Design review of the part built by this model. Coordinates are the model's own, in mm. Give positions to 0.01 mm unless a question says otherwise; leave off trailing zeros. Loops run counter-clockwise (first coordinate to the right, second up) from the corner with the lowest first, then second, coordinate; pieces in that order, holes last. Notation, with made-up numbers: (21, 4) - (66, 4) arc R19 ccw to (66, 23) - close; hole circle Ø2 at (-19.75, -38). An arc over 180 degrees is marked (long way). Write each question's results on one line, items separated by ' | '.
```python
from build123d import *

# Parameters (mm, degrees)
BOSS_EXTRUDE4_DEPTH  = 3.175
M3_CLEARANCE_HOLE3_D = 3
M3_CLEARANCE_HOLE1_D = 3.1
M3_CLEARANCE_HOLE4_D = 2.95
M3_CLEARANCE_HOLE2_D = 3.1
CUT_EXTRUDE1_DEPTH   = 121.250075364
BOSS_EXTRUDE6_DEPTH  = 3.175
CUT_EXTRUDE3_DEPTH   = 121.250075364
SKETCH25_R           = 1.5
CUT_EXTRUDE4_DEPTH   = 121.250075364


with BuildPart() as part:
    # Sketch1 → Boss-Extrude4 (new body)
    with BuildSketch(Plane(origin=(0, 0, 0), x_dir=(1, 0, 0), z_dir=(0, 1, 0))):
        with BuildLine():
            Line((-62.799553621, 32.496136604), (-73.969425011, 32.691107434))
            Line((-73.969425011, 32.691107434), (-77.053684287, 35.88495141))
            ThreePointArc((-77.053684287, 35.88495141), (-84.36642289, 10.358894189), (-83.446216027, -16.178041625))
            Line((-83.446216027, -16.178041625), (-79.680911643, -13.825218315))
            Line((-79.680911643, -13.825218315), (-69.484649137, -16.179210996))
            Line((-69.484649137, -16.179210996), (-43.094490772, -58.412292655))
            Line((-43.094490772, -58.412292655), (-43.094490772, -64.826600275))
            Line((-43.094490772, -64.826600275), (-34, -64.826600275))
            Line((-34, -64.826600275), (-34, -58.55))
            Line((-34, -58.55), (34, -58.55))
            Line((34, -58.55), (34, -64.826600275))
            Line((34, -64.826600275), (43.094490772, -64.826600275))
            Line((43.094490772, -64.826600275), (43.094490772, -58.412292655))
            Line((43.094490772, -58.412292655), (69.484649137, -16.179210996))
            Line((69.484649137, -16.179210996), (79.680911643, -13.825218315))
            Line((79.680911643, -13.825218315), (83.446216027, -16.178041625))
            ThreePointArc((83.446216027, -16.178041625), (84.36642289, 10.358894189), (77.053684287, 35.88495141))
            Line((77.053684287, 35.88495141), (73.969425011, 32.691107434))
            Line((73.969425011, 32.691107434), (62.799553621, 32.496136604))
            Line((62.799553621, 32.496136604), (30.284668021, 63.895396642))
            Line((30.284668021, 63.895396642), (30.089697191, 75.065268032))
            Line((30.089697191, 75.065268032), (33.173956467, 78.259112008))
            ThreePointArc((33.173956467, 78.259112008), (0, 85), (-33.173956467, 78.259112008))
            Line((-33.173956467, 78.259112008), (-30.089697191, 75.065268032))
            Line((-30.089697191, 75.065268032), (-30.284668021, 63.895396642))
            Line((-30.284668021, 63.895396642), (-62.799553621, 32.496136604))
        make_face()
    extrude(amount=BOSS_EXTRUDE4_DEPTH)

    # M3 Clearance Hole3 (through all)
    with Locations(Plane(origin=(0, 0, 0), x_dir=(-1, 0, 0), z_dir=(0, -1, 0))):
        with Locations((36.415, -50), (36.415, -38), (-36.415, -50), (-36.415, -38)):
            Hole(M3_CLEARANCE_HOLE3_D / 2)

    # M3 Clearance Hole1 (through all)
    with Locations(Plane(origin=(0, 3.175, 0), x_dir=(1, 0, 0), z_dir=(0, 1, 0))):
        with Locations((-78.542321426, -8.49139241), (78.542321426, -8.49139241), (74.155025063, 27.240269049), (-74.155025063, 27.240269049)):
            Hole(M3_CLEARANCE_HOLE1_D / 2)

    # M3 Clearance Hole4 (through all)
    with Locations(Plane(origin=(0, 0, 0), x_dir=(-1, 0, 0), z_dir=(0, -1, 0))):
        with Locations((-67.099301622, -15.278865202), (-50.141885166, -42.416404279), (-61.062544382, 30.698137949), (-38.043670771, 52.927205804), (50.141885166, -42.416404279), (67.099301622, -15.278865202), (38.043670771, 52.927205804), (61.062544382, 30.698137949)):
            Hole(M3_CLEARANCE_HOLE4_D / 2)

    # M3 Clearance Hole2 (through all)
    with Locations(Plane(origin=(0, 3.175, 0), x_dir=(1, 0, 0), z_dir=(0, 1, 0))):
        with Locations((27, 76.497766718), (-27, 76.497766718)):
            Hole(M3_CLEARANCE_HOLE2_D / 2)

    # Sketch20 → Cut-Extrude1 (cut, through all)
    with BuildSketch(Plane(origin=(0, 3.175, 0), x_dir=(1, 0, 0), z_dir=(0, 1, 0))):
        with BuildLine():
            Line((-14.64850035, 45.5), (-14.64850035, 40.5))
            ThreePointArc((-14.64850035, 40.5), (-16.14850035, 39), (-17.64850035, 40.5))
            Line((-17.64850035, 40.5), (-17.64850035, 45.5))
            ThreePointArc((-17.64850035, 45.5), (-16.14850035, 47), (-14.64850035, 45.5))
        make_face()
        with BuildLine():
            Line((14.64850035, 45.5), (14.64850035, 40.5))
            ThreePointArc((14.64850035, 40.5), (16.14850035, 39), (17.64850035, 40.5))
            Line((17.64850035, 40.5), (17.64850035, 45.5))
            ThreePointArc((17.64850035, 45.5), (16.14850035, 47), (14.64850035, 45.5))
        make_face()
    extrude(amount=-CUT_EXTRUDE1_DEPTH, mode=Mode.SUBTRACT)

    # Sketch22 → Boss-Extrude6 (add)
    with BuildSketch(Plane(origin=(0, 3.175, 0), x_dir=(1, 0, 0), z_dir=(0, 1, 0))):
        Polygon((-30.284668021, 63.895396642), (-30.245177733, 66.157793715), (-65.061950694, 32.535626892), (-62.799553621, 32.496136604), align=None)
        Polygon((-69.484649137, -16.179210996), (-71.689396914, -15.670204865), (-43.094490772, -61.431620518), (-43.094490772, -58.412292655), align=None)
        Polygon((43.094490772, -61.431620518), (71.689396914, -15.670204865), (69.484649137, -16.179210996), (43.094490772, -58.412292655), align=None)
        Polygon((65.061950694, 32.535626892), (30.245177733, 66.157793715), (30.284668021, 63.895396642), (62.799553621, 32.496136604), align=None)
    extrude(amount=-BOSS_EXTRUDE6_DEPTH)

    # Sketch24 → Cut-Extrude3 (cut, through all)
    with BuildSketch(Plane(origin=(0, 3.175, 0), x_dir=(1, 0, 0), z_dir=(0, 1, 0))):
        Polygon((-27, -52.75), (-27, -22.75), (-21.2, -22.75), (-21.2, 1.45), (0, 1.45), (21.2, 1.45), (21.2, -22.75), (27, -22.75), (27, -52.75), (21.2, -52.75), (21.2, -58.55), (-21.2, -58.55), (-21.2, -52.75), align=None)
    extrude(amount=-CUT_EXTRUDE3_DEPTH, mode=Mode.SUBTRACT)

    # Sketch25 → Cut-Extrude4 (cut, through all)
    with BuildSketch(Plane(origin=(0, 3.175, 0), x_dir=(1, 0, 0), z_dir=(0, 1, 0))):
        with Locations(Location((-24.1, -55.65, 0), (0, 0, 270))):
            Circle(SKETCH25_R)
        with Locations(Location((-24.1, -19.85, 0), (0, 0, 270))):
            Circle(SKETCH25_R)
        with Locations(Location((24.1, -19.85, 0), (0, 0, 270))):
            Circle(SKETCH25_R)
        with Locations(Location((24.1, -55.65, 0), (0, 0, 270))):
            Circle(SKETCH25_R)
    extrude(amount=-CUT_EXTRUDE4_DEPTH, mode=Mode.SUBTRACT)


solid = part.part
```
Item 1: We need section A-A on z = 29. Give the boundary of the cut face in (x, y) (3 decimals).
Output values:
outline: (-63.36, 0) - (-27, 0) - (-27, 3.175) - (-63.36, 3.175) - close; (27, 0) - (63.36, 0) - (63.36, 3.175) - (27, 3.175) - close
Item 2: Wall thickness on probe 1 along Z at (x, y) = (-37.5, 0.25); probe 2 along X at (y, z) = (2.9, -26); probe 3 along X at (y, z) = (1.25, 27): over which ranges is each line inside the solid? List them lowest first.
Output values:
probe 1: z = -59.15 to -54.3, -51.56 to 36.96, 39.04 to 48.96, 51.04 to 64.83 | probe 2: x = -80.93 to -75.08, -73.23 to 73.23, 75.08 to 80.93 | probe 3: x = -64.61 to -27, 27 to 64.61
Item 3: We need section B-B on x = 54. Give the boundary of the cut face in (y, z) (3 decimals).
Output values:
outline: (0, -43.218) - (3.175, -43.218) - (3.175, 43.979) - (0, 43.979) - close
Item 4: Clearance check with flat-ended pins moving along their axes: P1, Ø1, axis at y = 1.5, z = 14.5, coming from the +X side; P2, Ø1.6, axis at x = 25, y = 2, coming from the +Z side; P3, Ø1.6, axis at y = 2, z = -44, coming from the -X side. State where each tip first meets the part, or that it passes through.
Output values:
P1: stops at x = 83.84 | P2: stops at z = 58.55 | P3: stops at x = -54.02
Item 5: We need section D-D on x = -12. Give the boundary of the cut face in (y, z) (3 decimals).
Output values:
outline: (0, -84.149) - (3.175, -84.149) - (3.175, -1.45) - (0, -1.45) - close
Item 6: We need section C-C on y = 2.3. Give the number of separate pieces and of enclosed holes in the cut face, then the cut area to 3 significant figures.
Output values:
separate pieces: 1 | enclosed holes: 24 | area: 14,300 mm²
